Autodesk Inventor part; units mm, degrees
ref_plane "YZ Plane" through (0, 0, 0) normal (1, 0, 0) x (0, 1, 0)
ref_plane "XZ Plane" through (0, 0, 0) normal (0, 1, 0) x (-1, 0, 0)
ref_plane "XY Plane" through (0, 0, 0) normal (0, 0, 1) x (1, 0, 0)
sketch "Sketch1" plane through (0, 0, 0) normal (0, 1, 0) x (-1, 0, 0)
  line L0 (54, -67.5) -> (-54, -67.5)
  line L1 (-54, -67.5) -> (-54, 67.5)
  line L2 (-54, 67.5) -> (54, 67.5)
  line L3 (54, 67.5) -> (54, -67.5)
  line L4 (0, -94.5) -> (0, 94.5) construction
  line L5 (-75.6, 0) -> (75.6, 0) construction
  point P0 (0, 0)
  dimension "d0" = 108
  dimension "d1" = 135
extrude "Extrusion1" add sketch "Sketch1" along normal blind 10
sketch "Sketch2" plane through (-54, 0, 67.5) normal (0, 0, 1) x (1, 0, 0)
  line L0 (108, 10) -> (0, 10)
  line L1 (54, 10) -> (54, 0) construction
  line L2 (3.9342, 5) -> (111.9342, 5) construction
  point P0 (54, 5)
  point P1 (81, 5)
  point P2 (27, 5)
  dimension "d4" = 54
hole "Hole1" at (0, 5, 67.5) at (27, 5, 67.5) at (-27, 5, 67.5) direction (0, 0, -1) diameter 4.134 depth 14.2 tip angle 118
sketch "Sketch3" plane through (54, 0, -67.5) normal (0, 0, -1) x (-1, 0, 0)
  point P0 (54, 0)
  point P1 (27, 5)
  point P2 (54, 5)
  point P3 (81, 5)
hole "Hole2" at (27, 5, -67.5) at (0, 5, -67.5) at (-27, 5, -67.5) direction (0, 0, 1) diameter 4.134 depth 14.2 tip angle 118
properties part number "motor_base_plate" material "Aluminum 6061"
CAD build for the part. Positions are in the model's coordinates, mm. A direction names the side the tool comes from. Round coordinates to 2 decimals unless told otherwise and drop trailing zeros. One line per question, with ' | ' between items. Start each with the question number.
Item 1: Which spindle directions (+Z, -Z, +X, -X, +Y, -Y) get a long thin tool onto all of the face, cutting with end or side? Do faces 1 (the cylindrical face through (29.018, 5.448, 60.301)), 2 (the flat face through (1, 3, 67.5)), 3 (the cylindrical face through (-24.982, 4.552, -60.301)). Say none if no direction does.
Item 2: Pin check, flat tip, straight feed: pin 1 Ø2.5 at (x, y) = (27, 5) entering from -Z. Stop position of the tip, or through.
Item 3: Wall check: line 1 (X direction, y = 5, z = 59); line 2 (Y direction, x = -27, z = 60.25). Give the ranges that are in metal, low to high.
Responses:
1) face 1: +Z | face 2: +Z, +X, -X, +Y, -Y | face 3: -Z
2) pin 1: stops at z = -52.81
3) line 1: x = -54 to -29.07, -24.93 to -2.07, 2.07 to 24.93, 29.07 to 54 | line 2: y = 0 to 2.93, 7.07 to 10
